from build123d import *

# Parameters (mm, degrees)
SKETCH_1_R          = 6.5
EXTRUDE_1_DEPTH     = 1.7
EXTRUDE_2_DEPTH     = 4.2
SKETCH_3_R          = 2.5
CUT_EXTRUDE_1_DEPTH = 11.9229117


with BuildPart() as part:
    # Эскиз1 → Бобышка-Вытянуть1 (new body)
    with BuildSketch(Plane.XY):
        Circle(SKETCH_1_R)
    extrude(amount=EXTRUDE_1_DEPTH)

    # Эскиз2 → Бобышка-Вытянуть2 (add)
    with BuildSketch(Plane.XY.offset(1.7)):
        Polygon((5.773502692, 0), (2.886751346, 5), (-2.886751346, 5), (-5.773502692, 0), (-2.886751346, -5), (2.886751346, -5), align=None)
    extrude(amount=EXTRUDE_2_DEPTH)

    # Эскиз3 → Вырез-Вытянуть1 (cut, through all)
    with BuildSketch(Plane.XY.offset(5.9)):
        Circle(SKETCH_3_R)
    extrude(amount=-CUT_EXTRUDE_1_DEPTH, mode=Mode.SUBTRACT)


solid = part.part
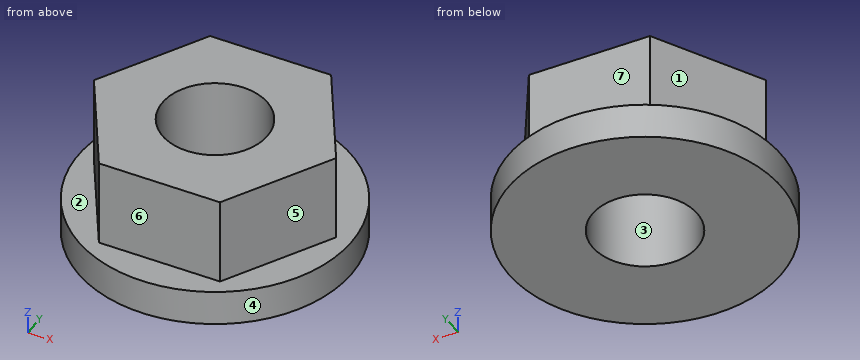
Input: part model. Units: mm. Frame: model coordinates. Face numbers are marked on the shaded views. A direction names the side the tool comes from. Coordinates: 2 decimals unless noted, no trailing zeros. Loops run counter-clockwise (first coordinate to the right, second up) from the corner with the lowest first, then second, coordinate; pieces in that order, holes last.
Q1. Set-up query: the marked faces 5, 6 and 7. Return all of +Z, -Z, +X, -X, +Y, -Y with unobstructed straight access to the full face (end or side cutting, diameter ignored); none if empty.
Q2. Cut plane B-B (z = 3.9). Output: boundary loops of the cut face in (x, y), then the cut area to 3 significant figures.
Q3. Material intervals for line 1 (Y direction, x = 0, z = 4); line 2 (Z direction, x = 4.25, y = 4.25); line 3 (Y direction, x = -2, z = 4), sorted ascending.
Q4. Contact query for flat-ended pins moving along their axis: pin 1 (2 mm diameter, centred on y = -3, z = 0.5, fed in from -X); pin 2 (6.5 mm diameter, centred on x = 0, y = 0, fed in from +Z); pin 3 (1 mm diameter, centred on y = -4, z = 3.5, fed in from +X); pin 4 (2 mm diameter, centred on x = 0.5, z = 3, fed in from +Y). Output: stop coordinate, or through.
Q5. Cut plane A-A (x = 0). Output: boundary loops of the cut face in (y, z).
Q6. Draft query along X for the marked faces 1, 2, 3 and 4. Return one class per face: +X half, -X half, draft (parallel to the pull), parting line (faces both ways), or undercut.
Q7. Cut plane C-C (y = 1.5). Output: boundary loops of the cut face in (x, z), then the cut area to 3 significant figures.
Q8. Cut plane D-D (x = -4.25). Output: boundary loops of the cut face in (y, z).
Working result:
1. face 5: +Z, +X, -Y
1. face 6: +Z, +X, -X, -Y
1. face 7: +Z, +X, -X, +Y
2. outline: (-5.77, 0) - (-2.89, -5) - (2.89, -5) - (5.77, 0) - (2.89, 5) - (-2.89, 5) - close; hole circle Ø5 at (0, 0)
2. area: 67.0 mm2
3. line 1: y = -5 to -2.5, 2.5 to 5
3. line 2: z = 0 to 1.7
3. line 3: y = -5 to -1.5, 1.5 to 5
4. pin 1: stops at x = -6.18
4. pin 2: stops at z = 5.9
4. pin 3: stops at x = 3.75
4. pin 4: stops at y = 5
5. outline: (-6.5, 0) - (-2.5, 0) - (-2.5, 5.9) - (-5, 5.9) - (-5, 1.7) - (-6.5, 1.7) - close; (2.5, 0) - (6.5, 0) - (6.5, 1.7) - (5, 1.7) - (5, 5.9) - (2.5, 5.9) - close
6. face 1: -X half
6. face 2: draft
6. face 3: undercut
6. face 4: parting line
7. outline: (-6.32, 0) - (-2, 0) - (-2, 5.9) - (-4.91, 5.9) - (-4.91, 1.7) - (-6.32, 1.7) - close; (2, 0) - (6.32, 0) - (6.32, 1.7) - (4.91, 1.7) - (4.91, 5.9) - (2, 5.9) - close
7. area: 39.1 mm2
8. outline: (-4.92, 0) - (4.92, 0) - (4.92, 1.7) - (2.64, 1.7) - (2.64, 5.9) - (-2.64, 5.9) - (-2.64, 1.7) - (-4.92, 1.7) - close
